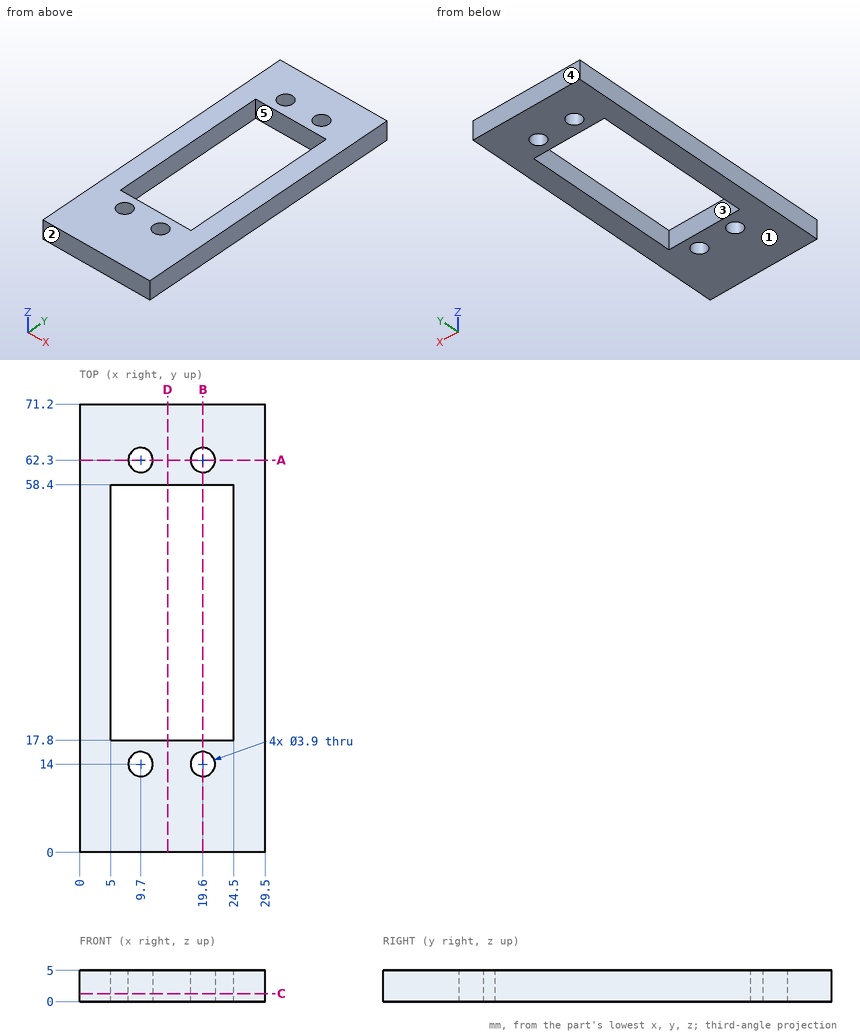
Verification items for this drawing (mm, ordinates from the low corner). A direction names the side the tool comes from. Round coordinates to 2 decimals unless told otherwise and drop trailing zeros. Write each loop counter-clockwise with the first axis right and the second up, starting at its lowest first coordinate (ties: lowest second). Pieces come first, ordered by that corner, then holes. Notation, with made-up numbers: (54.25, 3.5) - (78.25, 3.5) arc R24 cw to (78.25, 27.5) - close; hole circle Ø4 at (6.25, 12). An arc over 180 degrees is marked (long way). One line per item, written item: value.
1. Cross-section at D-D on x = 14. Record the boundary of the cut face in (y, z), and give its area (3 significant figures).
The answers:
outline: (0, 0) - (17.8, 0) - (17.8, 5) - (0, 5) - close; (58.4, 0) - (71.2, 0) - (71.2, 5) - (58.4, 5) - close
area: 153 mm^2
2. Cross-section at C-C on z = 1.3. Record the boundary of the cut face in (x, y).
The answers:
outline: (0, 0) - (29.5, 0) - (29.5, 71.2) - (0, 71.2) - close; hole (5, 17.8) - (24.5, 17.8) - (24.5, 58.4) - (5, 58.4) - close; hole circle Ø3.9 at (9.7, 14); hole circle Ø3.9 at (9.7, 62.3); hole circle Ø3.9 at (19.6, 14); hole circle Ø3.9 at (19.6, 62.3)
3. Depth check by flat-ended pin: pin 1 Ø6 at (x, y) = (19.6, 62.3) entering from -Z; pin 2 Ø3 at (x, y) = (19.6, 14) entering from -Z. Enter the tip coordinate at first touch or a pass-through.
The answers:
pin 1: stops at z = 0
pin 2: passes through
4. Scan lines: L1, parallel to Y at x = 19.6, z = 2.05; L2, parallel to X at y = 20, z = 3.3; L3, parallel to Y at x = 10.5, z = 4.7. Record each from-to range of solid material in increasing order.
The answers:
L1: y = 0 to 12.05, 15.95 to 17.8, 58.4 to 60.35, 64.25 to 71.2
L2: x = 0 to 5, 24.5 to 29.5
L3: y = 0 to 12.22, 15.78 to 17.8, 58.4 to 60.52, 64.08 to 71.2
5. Set-up check for the marked faces 4 and 5: record each of +Z, -Z, +X, -X, +Y, -Y from which the full face is reachable in a straight line by a thin tool's end or side.
The answers:
face 4: +Z, -Z, +X, -X, +Y
face 5: +Z, -Z
6. Mould release check, pull along Y, two halves, no side actions. Record for the marked faces 1, 2 and 3: released by +Y, released by -Y, zero draft, split by the parting line, or undercut.
The answers:
face 1: zero draft
face 2: released by -Y
face 3: undercut
7. Cross-section at B-B on x = 19.6. Record the boundary of the cut face in (y, z), and give its area (3 significant figures).
The answers:
outline: (0, 0) - (12.05, 0) - (12.05, 5) - (0, 5) - close; (15.95, 0) - (17.8, 0) - (17.8, 5) - (15.95, 5) - close; (58.4, 0) - (60.35, 0) - (60.35, 5) - (58.4, 5) - close; (64.25, 0) - (71.2, 0) - (71.2, 5) - (64.25, 5) - close
area: 114 mm^2
8. Cross-section at A-A on y = 62.3. Record the boundary of the cut face in (x, z), and give its area (4 significant figures).
The answers:
outline: (0, 0) - (7.75, 0) - (7.75, 5) - (0, 5) - close; (11.65, 0) - (17.65, 0) - (17.65, 5) - (11.65, 5) - close; (21.55, 0) - (29.5, 0) - (29.5, 5) - (21.55, 5) - close
area: 108.5 mm^2
